The listing builds one solid part. Answer for the finished solid, in the listing's coordinates (mm). A direction names the side the tool comes from. Round coordinates to 2 decimals unless told otherwise and drop trailing zeros. Order: outer loops, then holes, each group sorted by start corner. A loop starts at its lowest first (then second) coordinate and runs counter-clockwise, first axis right, second up. Notation, with made-up numbers: (12, 10.5) - (26, 10.5) arc R23 cw to (26, 31.5) - close; hole circle Ø4 at (38, 63.25). An arc over 180 degrees is marked (long way). Use CSV: the item, a comma, the result in double quotes. Start each with the question number.
Item 1: Straight lines are drawn through the part: line 1 along Z through (x, y) = (14, -13); line 2 along X through (y, z) = (375.5, -28.5); line 3 along Z through (x, y) = (23.5, 28). For each, find the intervals that lie inside material, in ascending order. Write a range as [from, to].
Item 2: Find section A-A, the plane z = -14.5. Give the vertices of the cut face in (x, y), plus the area to 3 significant figures.
Item 3: Determine the mould class of faces 3 (the flat face through (26, 258, -44.45)), 4 (the flat face through (36, 258, -50.8)), 5 (the flat face through (50.8, 258, -26)) for opening direction X: +X half, -X half, draft (parallel to the pull), parting line (faces both ways), or undercut.
Item 4: Find section B-B, the plane y = 448. Give the vertices of the cut face in (x, z) (3 decimals).
Item 5: For faces 1 (the flat face through (25, 258, 0)), 2 (the flat face through (44.45, 258, -25)), determine the directions among +Z, -Z, +X, -X, +Y, -Y from which every point of the face is accessible in a straight line to the end or side of a thin tool.
Item 6: Flat-ended cylindrical pins translate along their axes: P1, Ø1.9, axis at x = 24.5, y = 256, coming from the -Z side; P2, Ø0.8, axis at y = 377, z = -49, coming from the +X side; P3, Ø0.8, axis at y = 405, z = -49.5, coming from the -X side. Find the tip coordinate at first contact, or state that the pin passes through.
```python
from build123d import *

# Parameters (mm, degrees)
SKETCH1_W           = 50.8
SKETCH1_H           = 50.8
BOSS_EXTRUDE1_DEPTH = 558.8
SKETCH3_W           = 50.8
SKETCH3_H           = 50.8
BOSS_EXTRUDE2_DEPTH = 50.8
FILLET2_R           = 6.35
SKETCH4_W           = 6.35
SKETCH4_H           = 609.6
CUT_EXTRUDE2_DEPTH  = 2.54
CUT_EXTRUDE3_DEPTH  = 614.818735459


with BuildPart() as part:
    # Sketch1 → Boss-Extrude1 (new body)
    with BuildSketch(Plane(origin=(0, 0, 0), x_dir=(1, 0, 0), z_dir=(0, 1, 0))):
        with Locations((25.4, 25.4)):
            Rectangle(SKETCH1_W, SKETCH1_H)
    extrude(amount=BOSS_EXTRUDE1_DEPTH)

    # Sketch3 → Boss-Extrude2 (add)
    with BuildSketch(Plane.XZ):
        with Locations((25.4, -25.4)):
            Rectangle(SKETCH3_W, SKETCH3_H)
    extrude(amount=BOSS_EXTRUDE2_DEPTH)

    # Fillet2
    fillet2_edges = [part.edges().sort_by_distance(p)[0] for p in [
        (0, 254, -50.8),
        (50.8, 254, -50.8),
        (50.8, 254, 0),
        (0, 254, 0),
    ]]
    fillet(fillet2_edges, radius=FILLET2_R)

    # Sketch4 → Cut-Extrude2 (cut)
    with BuildSketch(Plane(origin=(0, 0, -50.8), x_dir=(-1, 0, 0), z_dir=(0, 0, -1))):
        with Locations((-25.4, 254)):
            Rectangle(SKETCH4_W, SKETCH4_H)
    extrude(amount=-CUT_EXTRUDE2_DEPTH, mode=Mode.SUBTRACT)

    # Sketch5 → Cut-Extrude3 (cut, through all)
    with BuildSketch(Plane(origin=(0, 558.8, 0), x_dir=(1, 0, 0), z_dir=(0, 1, 0))):
        with BuildLine():
            Line((34.925, 44.45), (15.875, 44.45))
            Line((15.875, 44.45), (8.89, 44.45))
            ThreePointArc((8.89, 44.45), (7.093948776, 43.706051224), (6.35, 41.91))
            Line((6.35, 41.91), (6.35, 8.89))
            ThreePointArc((6.35, 8.89), (7.093948776, 7.093948776), (8.89, 6.35))
            Line((8.89, 6.35), (41.91, 6.35))
            ThreePointArc((41.91, 6.35), (43.706051224, 7.093948776), (44.45, 8.89))
            Line((44.45, 8.89), (44.45, 41.91))
            ThreePointArc((44.45, 41.91), (43.706051224, 43.706051224), (41.91, 44.45))
            Line((41.91, 44.45), (34.925, 44.45))
        make_face()
    extrude(amount=-CUT_EXTRUDE3_DEPTH, mode=Mode.SUBTRACT)


solid = part.part
```
Worked out:
1,line 1,"z = [-50.8, -44.45], [-6.35, 0]"
1,line 2,"x = [0, 6.35], [44.45, 50.8]"
1,line 3,"z = [-48.26, -44.45], [-6.35, 0]"
2,outline,"(0, -50.8) - (6.35, -50.8) - (6.35, 558.8) - (0, 558.8) - close; (44.45, -50.8) - (50.8, -50.8) - (50.8, 558.8) - (44.45, 558.8) - close"
2,area,"7,740 mm²"
3,face 3,"undercut"
3,face 4,"draft"
3,face 5,"+X half"
4,outline,"(0, -44.45) arc R6.35 ccw to (6.35, -50.8) - (22.225, -50.8) - (22.225, -48.26) - (28.575, -48.26) - (28.575, -50.8) - (44.45, -50.8) arc R6.35 ccw to (50.8, -44.45) - (50.8, -6.35) arc R6.35 ccw to (44.45, 0) - (6.35, 0) arc R6.35 ccw to (0, -6.35) - close; hole (6.35, -41.91) arc R2.54 ccw to (8.89, -44.45) - (41.91, -44.45) arc R2.54 ccw to (44.45, -41.91) - (44.45, -8.89) arc R2.54 ccw to (41.91, -6.35) - (8.89, -6.35) arc R2.54 ccw to (6.35, -8.89) - close"
5,face 1,"+Z, +X, -X, +Y, -Y"
5,face 2,"+Y, -Y"
6,P1,"stops at z = -48.26"
6,P2,"stops at x = 49.26"
6,P3,"stops at x = 2.03"
